Input: part model. Units: mm. Frame: model coordinates. A direction names the side the tool comes from. Round coordinates to 2 decimals unless told otherwise and drop trailing zeros. Order: outer loops, then holes, each group sorted by start corner. A loop starts at its lowest first (then second) coordinate and runs counter-clockwise, first axis right, second up.
Item 1: Mould query, pull axis Y, two halves, no side actions, for faces 4 (the flat face through (55.467, 25.606, 4.479)), 5 (the flat face through (70, 0, 3)), 6 (the flat face through (40, 27, 8)). Classes: released by +Y, released by -Y, zero draft, split by the parting line, or undercut.
Item 2: Line query: L1, parallel to Y at x = 52.75, z = 15.5; L2, parallel to X at y = -24.25, z = 15.25; L3, parallel to Z at x = 19, y = 11. Output: solid intervals per line, ascending.
Item 3: Cut plane D-D on z = 13. Output: boundary loops of the cut face in (x, y), then the cut area to 3 significant figures.
Item 4: Cut plane B-B on x = 48. Output: boundary loops of the cut face in (y, z), then the cut area to 3 significant figures.
Item 5: Reachability of faces 1 (the flat face through (35, -10, 0)), 2 (the flat face through (35, 19, 3)), 3 (the flat face through (55.36, 22.71, 4.48)) from +Z, -Z, +X, -X, +Y, -Y: full face, straight path, thin tool, end or side. Return the list, or none.
Item 6: Cut plane A-A on z = -4. Output: boundary loops of the cut face in (x, y), then the cut area to 3 significant figures.
Item 7: First-contact query: pin 1 (2 mm diameter, centred on x = 47.5, z = 20.5, fed in from +Y); pin 2 (2.5 mm diameter, centred on x = 52, z = 4.5, fed in from -Y); pin 3 (7 mm diameter, centred on x = 65.5, y = 11.5, fed in from +Z); pin 4 (9 mm diameter, centred on y = 8.5, z = 20, fed in from -X). Flat tips, straight axial feed; report the tip coordinate or a pass-through.
Item 8: Cut plane C-C on y = 1. Output: boundary loops of the cut face in (x, z).
Autodesk Inventor part; units mm, degrees
ref_plane "YZ Plane" through (0, 0, 0) normal (1, 0, 0) x (0, 1, 0)
ref_plane "XZ Plane" through (0, 0, 0) normal (0, 1, 0) x (-1, 0, 0)
ref_plane "XY Plane" through (0, 0, 0) normal (0, 0, 1) x (1, 0, 0)
sketch "Sketch2" plane through (0, 0, 0) normal (1, 0, 0) x (0, 1, 0)
  line L0 (-19.9252, 0) -> (19.9252, 0)
  line L1 (0, -28.9507) -> (0, 28.9507)
  line L2 (14.5, -7.3) -> (-14.5, -7.3)
  line L3 (-14.5, -7.3) -> (-14.5, -3)
  line L4 (-10, -3) -> (-10, 3)
  line L5 (-27, 3) -> (-27, 9)
  line L6 (-27, 9) -> (27, 9)
  line L7 (14.5, -7.3) -> (14.5, -3)
  line L8 (10, -3) -> (10, 3)
  line L9 (27, 3) -> (27, 9)
  line L10 (-14.5, -3) -> (-10, -3)
  line L11 (10, -3) -> (14.5, -3)
  line L12 (27, 3) -> (10, 3)
  line L13 (-10, 3) -> (-27, 3)
  point P0 (0, 0)
  point P1 (0, 0)
  point P2 (10, 0)
  dimension "d4" = 14.5
  dimension "d8" = 27
  dimension "d9" = 10
  dimension "d10" = 4.3
  dimension "d11" = 6
  dimension "d12" = 6
extrude "Extrusion2" add sketch "Sketch2" along normal blind 70
sketch "Sketch3" plane through (0, -27, 9) normal (0, 0, 1) x (1, 0, 0)
  line L0 (0, 0) -> (70, 0)
  line L1 (0, 54) -> (70, 54)
  line L2 (55.5, 0) -> (50, 0)
  line L3 (50, 0) -> (50, 54)
  line L4 (50, 54) -> (55.5, 54)
  line L5 (55.5, 54) -> (55.5, 0)
  line L6 (70, 54) -> (70, 0)
  point P0 (0, 27)
  dimension "d15" = 20
  dimension "d16" = 5.5
extrude "Extrusion3" add sketch "Sketch3" along normal blind 17 contours L3 L1 L5 L0
sketch "Sketch4" plane through (50, -27, 9) normal (-1, 0, 0) x (0, 0, 1)
  line L0 (17, 54) -> (17, 0)
  circle A0 centre (17, 42) radius 6.5
  circle A1 centre (17, 12) radius 6.5
  line L1 (0, 0) -> (17, 0)
  point P0 (-9, 27)
  dimension "d19" = 13
  dimension "d20" = 13
  dimension "d21" = 30
  dimension "d22" = 12
extrude "Extrusion4" cut sketch "Sketch4" against normal up to surface (5.5 mm away)
sketch "Sketch5" plane through (0, -14.5, -7.3) normal (0, 0, -1) x (-1, 0, 0)
  line L0 (0, 0) -> (-70, 0)
  line L1 (-55.5, 29) -> (-55.5, 0)
  line L2 (-50, 0) -> (-50, 29)
  line L3 (-50, 14.5) -> (-55.5, 14.5)
  line L4 (-50, -12.5) -> (-50, 41.5)
  line L5 (-55.5, 41.5) -> (-55.5, -12.5)
  line L6 (0, -12.5) -> (-70, -12.5)
  point P0 (0, 27)
  point P1 (-52.75, -9.75)
  point P2 (-52.75, 14.5)
  point P3 (-52.75, 38.75)
  dimension "d26" = 2.75
  dimension "d34" = 2.75
hole "Hole1" at (52.75, -24.25, -7.3) at (52.75, 0, -7.3) at (52.75, 24.25, -7.3) direction (0, 0, 1) diameter 4.5 end through all
sketch "Sketch6" plane through (0, -14.5, -7.3) normal (0, 0, -1) x (-1, 0, 0)
  circle A0 centre (-52.75, 14.5) radius 2.25
  line L0 (-56.25, 14.5) -> (-54.5, 17.5311)
  line L1 (-54.5, 17.5311) -> (-51, 17.5311)
  line L2 (-51, 17.5311) -> (-49.25, 14.5)
  line L3 (-49.25, 14.5) -> (-51, 11.4689)
  line L4 (-51, 11.4689) -> (-54.5, 11.4689)
  line L5 (-54.5, 11.4689) -> (-56.25, 14.5)
  circle A1 centre (-52.75, 38.75) radius 2.25
  line L6 (-56.25, 38.75) -> (-54.5, 41.7811)
  line L7 (-54.5, 41.7811) -> (-51, 41.7811)
  line L8 (-51, 41.7811) -> (-49.25, 38.75)
  line L9 (-49.25, 38.75) -> (-51, 35.7189)
  line L10 (-51, 35.7189) -> (-54.5, 35.7189)
  line L11 (-54.5, 35.7189) -> (-56.25, 38.75)
  circle A2 centre (-52.75, -9.75) radius 2.25
  line L12 (-56.25, -9.75) -> (-54.5, -6.7189)
  line L13 (-54.5, -6.7189) -> (-51, -6.7189)
  line L14 (-51, -6.7189) -> (-49.25, -9.75)
  line L15 (-49.25, -9.75) -> (-51, -12.7811)
  line L16 (-51, -12.7811) -> (-54.5, -12.7811)
  line L17 (-54.5, -12.7811) -> (-56.25, -9.75)
  point P0 (0, 14.5)
  dimension "d35" = 7
  dimension "d36" = 7
  dimension "d37" = 7
extrude "Extrusion5" cut sketch "Sketch6" against normal blind 13.3
chamfer "Chamfer1" distance 6 angle 45 2 edges at (50, 0, 9) (55.5, 0, 9)
equation "\"d23\" = d21"
properties part number "CarroXY - Hotend"
From the geometry:
1. face 4: undercut
1. face 5: zero draft
1. face 6: released by +Y
2. L1: y = -27 to -26.5, -22 to -2.25, 2.25 to 22, 26.5 to 27
2. L2: x = 50 to 50.5, 55 to 55.5
2. L3: z = -7.3 to -3, 3 to 9
3. outline: (48, -27) - (57.5, -27) - (57.5, 27) - (48, 27) - close; hole circle Ø4.5 at (52.75, -24.25); hole circle Ø4.5 at (52.75, 0); hole circle Ø4.5 at (52.75, 24.25)
3. area: 465 mm2
4. outline: (-27, 3) - (-10, 3) - (-10, -3) - (-14.5, -3) - (-14.5, -7.3) - (14.5, -7.3) - (14.5, -3) - (10, -3) - (10, 3) - (27, 3) - (27, 13) - (-27, 13) - close
4. area: 785 mm2
5. face 1: +X, -X, -Y
5. face 2: +X, -X, +Y
5. face 3: -Z
6. outline: (0, -14.5) - (70, -14.5) - (70, 14.5) - (0, 14.5) - close; hole (49.25, 0) - (51, -3.03) - (54.5, -3.03) - (56.25, 0) - (54.5, 3.03) - (51, 3.03) - close
6. area: 2,000 mm2
7. pin 1: passes through
7. pin 2: stops at y = -27
7. pin 3: stops at z = 9
7. pin 4: stops at x = 50
8. outline: (0, -7.3) - (49.83, -7.3) - (49.83, 6) - (50.73, 6) - (50.73, 26) - (50, 26) - (50, 15) - (44, 9) - (0, 9) - close; (54.77, 6) - (55.67, 6) - (55.67, -7.3) - (70, -7.3) - (70, 9) - (61.5, 9) - (55.5, 15) - (55.5, 26) - (54.77, 26) - close
